Could you check a few things on this model? Use its own coordinates, in mm. A direction names the side the tool comes from. Round coordinates to 2 decimals unless told otherwise and drop trailing zeros. Loops run counter-clockwise (first coordinate to the right, second up) from the corner with the lowest first, then second, coordinate; pieces in that order, holes last. Notation, with made-up numbers: (37, -20.5) -> (78, -20.5) arc R29 ccw to (78, 8.5) -> close; hole circle Ø10 at (21, 7.25). An arc over 180 degrees is marked (long way). Write each question's results on one line, items separated by ' | '.
from build123d import *

# Parameters (mm, degrees)
BOSS_EXTRUDE1_DEPTH  = 25
M3_CLEARANCE_HOLE1_D = 3.4
SKETCH6_R            = 7.89
CUT_EXTRUDE1_DEPTH   = 3
FILLET1_R            = 12.5
FILLET2_R            = 2
SKETCH7_R            = 12.5
SKETCH7_R_2          = 6.79
BOSS_EXTRUDE2_DEPTH  = 3
CUT_EXTRUDE2_START   = -5
SKETCH9_R            = 7.89
CUT_EXTRUDE2_DEPTH   = 5


with BuildPart() as part:
    # Sketch2 → Boss-Extrude1 (new body)
    with BuildSketch(Plane.XY):
        with BuildLine():
            Line((0, 63), (-25, 63))
            Line((-25, 63), (-25, 60))
            Line((-25, 60), (0, 60))
            ThreePointArc((0, 60), (42.611122537, 42.240883467), (59.997715384, -0.52359213))
            Line((59.997715384, -0.52359213), (59.779551996, -25.522640207))
            Line((59.779551996, -25.522640207), (62.779437766, -25.548819813))
            Line((62.779437766, -25.548819813), (62.997601153, -0.549771736))
            ThreePointArc((62.997601153, -0.549771736), (44.741678664, 44.352927641), (0, 63))
        make_face()
    extrude(amount=BOSS_EXTRUDE1_DEPTH)

    # M3 Clearance Hole1 (through all)
    with Locations(Plane(origin=(0, 63, 0), x_dir=(1, 0, 0), z_dir=(0, 1, 0))):
        with Locations((-20, -5), (-5, -20), (-20, -20), (-5, -5)):
            Hole(M3_CLEARANCE_HOLE1_D / 2)

    # Sketch6 → Cut-Extrude1 (cut)
    with BuildSketch(Plane(origin=(62.997601153, -0.549771736, 0), x_dir=(0, 0, -1), z_dir=(0.9999619230641714, -0.00872653549837746, 0))):
        with Locations(Location((-12.5, -12.5, 0), (0, 0, 90))):
            Circle(SKETCH6_R)
    extrude(amount=-CUT_EXTRUDE1_DEPTH, mode=Mode.SUBTRACT)

    # Fillet1
    fillet1_edges = [part.edges().sort_by_distance(p)[0] for p in [
        (61.279494881, -25.53573001, 0),
        (61.279494881, -25.53573001, 25),
    ]]
    fillet(fillet1_edges, radius=FILLET1_R - 0.0001)  # a hair under: the kernel refuses the full size

    # Fillet2
    fillet2_edges = [part.edges().sort_by_distance(p)[0] for p in [
        (-25, 61.5, 25),
        (-25, 61.5, 0),
    ]]
    fillet(fillet2_edges, radius=FILLET2_R)

    # Sketch7 → Boss-Extrude2 (add)
    with BuildSketch(Plane(origin=(62.997601153, -0.549771736, 0), x_dir=(0, 0, -1), z_dir=(0.9999619230641714, -0.00872653549837732, 0))):
        with Locations(Location((-12.5, -12.5, 0), (0, 0, 90))):
            Circle(SKETCH7_R)
        with Locations(Location((-12.5, -12.5, 0), (0, 0, 90))):
            Circle(SKETCH7_R_2, mode=Mode.SUBTRACT)
    extrude(amount=BOSS_EXTRUDE2_DEPTH)

    # Sketch9 → Cut-Extrude2 (cut)
    with BuildSketch(Plane(origin=(59.997715384, -0.52359213, 0), x_dir=(0, 0, 1), z_dir=(-0.9999619230641714, 0.008726535498377324, 0)).offset(CUT_EXTRUDE2_START)):
        with Locations(Location((12.5, -12.5, 0), (0, 0, 90))):
            Circle(SKETCH9_R)
    extrude(amount=CUT_EXTRUDE2_DEPTH, mode=Mode.SUBTRACT)


solid = part.part
1) If we mould it in two halves opening along Z, with no side actions, what happens to faces 1 (the flat face through (42, 45, 25)), 2 (the cylindrical face through (42.14, 42.71, 12.32)), 3 (the cylindrical face through (65.409, -9.938, 6.476))? For each: released by +Z, released by -Z, zero draft, split by the parting line, or undercut.
Model answer:
face 1: released by +Z | face 2: zero draft | face 3: undercut
2) I want a section at D-D, the plane x = 28. Write out the boundary of the cut face in (y, z), plus the area to 3 significant figures.
Model answer:
outline: (53.07, 0) -> (56.44, 0) -> (56.44, 25) -> (53.07, 25) -> close | area: 84.2 mm2
3) For faces 4 (the flat face through (-13, 60, 12)), 5 (the cylindrical face through (-20.914, 61.479, 18.567)), which set-ups out of +Z, -Z, +X, -X, +Y, -Y let a thin tool reach every point of the face, with its end or its side?
Model answer:
face 4: +Z, -Z, -X, -Y | face 5: +Y, -Y
4) I need wall thicknesses on line 1 (Z direction, x = -20, y = 62.2); line 2 (Y direction, x = -10, z = 24.25); line 3 (X direction, y = 7, z = 8.5). Which ranges of each line are inside material? Lowest first, please.
Model answer:
line 1: z = 0 to 3.3, 6.7 to 18.3, 21.7 to 25 | line 2: y = 60 to 63 | line 3: x = 59.59 to 62.61
5) I want a section at A-A, the plane x = -5. Write out the boundary of the cut face in (y, z).
Model answer:
outline: (60, 0) -> (63, 0) -> (63, 3.3) -> (60, 3.3) -> close; (60, 6.7) -> (63, 6.7) -> (63, 18.3) -> (60, 18.3) -> close; (60, 21.7) -> (63, 21.7) -> (63, 25) -> (60, 25) -> close
6) I'm going to push flat-ended pins straight in: pin 1 (6 mm diameter, centred on y = 40.5, z = 3.5, fed in from -X); pin 2 (1.5 mm diameter, centred on y = 35, z = 4.5, fed in from -X); pin 3 (4 mm diameter, centred on x = -3, z = 8, fed in from -Y). Where does each tip first touch, or does it pass through?
Model answer:
pin 1: stops at x = 41.32 | pin 2: stops at x = 48.19 | pin 3: stops at y = 60
7) I want a section at B-B, the plane z = 11. Write out the boundary of the cut face in (x, y), plus the area to 3 significant figures.
Model answer:
outline: (-25, 60) -> (0, 60) arc R60 cw to (60, -0.52) -> (59.96, -5.28) -> (64.96, -5.32) -> (64.95, -6.44) -> (65.95, -6.45) -> (66, -0.67) -> (63, -0.64) -> (63, -0.55) arc R63 ccw to (0, 63) -> (-25, 63) -> close; (59.78, -25.43) -> (65.78, -25.48) -> (65.83, -19.7) -> (64.83, -19.69) -> (64.82, -20.81) -> (59.82, -20.77) -> close | area: 425 mm2
8) I want a section at C-C, the plane y = 31.5. Write out the boundary of the cut face in (x, z), plus the area to 3 significant figures.
Model answer:
outline: (51.07, 0) -> (54.56, 0) -> (54.56, 25) -> (51.07, 25) -> close | area: 87.3 mm2
